```python
from build123d import *

# Parameters (mm, degrees)
SKETCH1_W                      = 1625.6
SKETCH1_H                      = 63.5
BASE_FLANGE1_DEPTH             = 1.89738
EDGE_FLANGE1_STRIP_W           = 12.66952
EDGE_FLANGE1_STRIP_H           = 1.89738
EDGE_FLANGE1_STRIP_CUT_DEPTH   = 1625.6
EDGE_FLANGE1_STRIP_2_W         = 12.66952
EDGE_FLANGE1_STRIP_2_H         = 1.89738
EDGE_FLANGE1_STRIP_CUT_2_DEPTH = 1625.6
EDGE_FLANGE1_DEPTH             = 1625.6
EDGE_FLANGE1_BEND_DEPTH        = 1625.6
SKETCH15_W                     = 9.525
SKETCH15_H                     = 50.8
CUT_EXTRUDE2_DEPTH             = 4.7752
LPATTERN3_COUNT                = 4
LPATTERN3_PITCH                = 457.2
SKETCH16_R                     = 3.3655
CUT_EXTRUDE3_DEPTH             = 2.54
LPATTERN4_COUNT                = 3
LPATTERN4_PITCH                = 762
CUT_EXTRUDE4_DEPTH             = 2.54
LPATTERN5_COUNT                = 2
LPATTERN5_PITCH                = 736.6
SKETCH18_R                     = 2.4638
CUT_EXTRUDE5_DEPTH             = 1628.038035818
SKETCH19_R                     = 2.4638
CUT_EXTRUDE6_DEPTH             = 1628.038035818
CHAMFER1_SIZE                  = 2.54


# Sheet-metal steps are written as plain solids
with BuildPart() as part:
    # Sketch1 → Base-Flange1 (new body)
    with BuildSketch(Plane(origin=(0, 0, 0), x_dir=(0, 0, -1), z_dir=(1, 0, 0))):
        with Locations((812.8, 31.75)):
            Rectangle(SKETCH1_W, SKETCH1_H)
    extrude(amount=-BASE_FLANGE1_DEPTH)

    # Edge-Flange1 strip (across the edge) → Edge-Flange1 strip cut (cut)
    with BuildSketch(Plane(origin=(-1.89738, 63.5, 0), x_dir=(0, -1, 0), z_dir=(0, 0, -1))):
        with Locations((-1.89738, -0.94869)):
            Rectangle(EDGE_FLANGE1_STRIP_W, EDGE_FLANGE1_STRIP_H)
    extrude(amount=EDGE_FLANGE1_STRIP_CUT_DEPTH, mode=Mode.SUBTRACT)

    # Edge-Flange1 strip 2 (across the edge) → Edge-Flange1 strip cut 2 (cut)
    with BuildSketch(Plane(origin=(-1.89738, 0, -1625.6), x_dir=(0, 1, 0), z_dir=(0, 0, 1))):
        with Locations((-1.89738, -0.94869)):
            Rectangle(EDGE_FLANGE1_STRIP_2_W, EDGE_FLANGE1_STRIP_2_H)
    extrude(amount=EDGE_FLANGE1_STRIP_CUT_2_DEPTH, mode=Mode.SUBTRACT)

    # Edge-Flange1 section (across the edge) → Edge-Flange1 (add)
    with BuildSketch(Plane(origin=(-1.89738, 63.5, 0), x_dir=(0, -1, 0), z_dir=(0, 0, -1))):
        with BuildLine():
            Line((0, 2.54), (0, 23.50262))
            Line((0, 23.50262), (1.89738, 23.50262))
            Line((1.89738, 23.50262), (1.89738, 2.54))
            ThreePointArc((1.89738, 2.54), (2.641328776, 0.743948776), (4.43738, 0))
            Line((4.43738, 0), (4.43738, -1.89738))
            ThreePointArc((4.43738, -1.89738), (1.299678511, -0.597701489), (0, 2.54))
        make_face()
    extrude(amount=EDGE_FLANGE1_DEPTH)

    # Edge-Flange1 section 2 (across the edge) → Edge-Flange1 bend (add)
    with BuildSketch(Plane(origin=(-1.89738, 0, -1625.6), x_dir=(0, 1, 0), z_dir=(0, 0, 1))):
        with BuildLine():
            Line((0, 2.54), (0, 23.50262))
            Line((0, 23.50262), (1.89738, 23.50262))
            Line((1.89738, 23.50262), (1.89738, 2.54))
            ThreePointArc((1.89738, 2.54), (2.641328776, 0.743948776), (4.43738, 0))
            Line((4.43738, 0), (4.43738, -1.89738))
            ThreePointArc((4.43738, -1.89738), (1.299678511, -0.597701489), (0, 2.54))
        make_face()
    extrude(amount=EDGE_FLANGE1_BEND_DEPTH)

    # Sketch15 → Cut-Extrude2 (cut)
    with BuildSketch(Plane(origin=(0, 63.5, 0), x_dir=(1, 0, 0), z_dir=(0, 1, 0))):
        with Locations((-4.7625, 127)):
            Rectangle(SKETCH15_W, SKETCH15_H)
    cut_extrude2 = extrude(amount=-CUT_EXTRUDE2_DEPTH, mode=Mode.SUBTRACT)

    # LPattern3: Cut-Extrude2 ×4
    with Locations(*[(0, 0, -i * LPATTERN3_PITCH) for i in range(1, LPATTERN3_COUNT)]):
        add(cut_extrude2, mode=Mode.SUBTRACT)

    # Sketch16 → Cut-Extrude3 (cut)
    with BuildSketch(Plane(origin=(0, 63.5, 0), x_dir=(1, 0, 0), z_dir=(0, 1, 0))):
        with Locations(Location((-12.7, 1574.8, 0), (0, 0, 180))):
            Circle(SKETCH16_R)
    cut_extrude3 = extrude(amount=-CUT_EXTRUDE3_DEPTH, mode=Mode.SUBTRACT)

    # LPattern4: Cut-Extrude3 ×3
    with Locations(*[(0, 0, i * LPATTERN4_PITCH) for i in range(1, LPATTERN4_COUNT)]):
        add(cut_extrude3, mode=Mode.SUBTRACT)

    # Sketch17 → Cut-Extrude4 (cut)
    with BuildSketch(Plane(origin=(0, 0, 0), x_dir=(0, 0, -1), z_dir=(1, 0, 0))):
        with BuildLine():
            Line((381, 47.625), (508, 47.625))
            ThreePointArc((508, 47.625), (523.875, 31.75), (508, 15.875))
            Line((508, 15.875), (381, 15.875))
            ThreePointArc((381, 15.875), (365.125, 31.75), (381, 47.625))
        make_face()
    cut_extrude4 = extrude(amount=-CUT_EXTRUDE4_DEPTH, mode=Mode.SUBTRACT)

    # LPattern5: Cut-Extrude4 ×2
    with Locations(*[(0, 0, -i * LPATTERN5_PITCH) for i in range(1, LPATTERN5_COUNT)]):
        add(cut_extrude4, mode=Mode.SUBTRACT)

    # Sketch18 → Cut-Extrude5 (cut, through all)
    with BuildSketch(Plane(origin=(0, 0, 0), x_dir=(0, 0, -1), z_dir=(1, 0, 0))):
        with Locations((546.1, 50.8)):
            Circle(SKETCH18_R)
        with Locations((546.1, 12.7)):
            Circle(SKETCH18_R)
    cut_extrude5 = extrude(amount=-CUT_EXTRUDE5_DEPTH, mode=Mode.SUBTRACT)

    # Sketch19 → Cut-Extrude6 (cut, through all)
    with BuildSketch(Plane(origin=(0, 0, 0), x_dir=(0, 0, -1), z_dir=(1, 0, 0))):
        with Locations((12.7, 50.8)):
            Circle(SKETCH19_R)
        with Locations((12.7, 12.7)):
            Circle(SKETCH19_R)
    cut_extrude6 = extrude(amount=-CUT_EXTRUDE6_DEPTH, mode=Mode.SUBTRACT)

    # Mirror1: Cut-Extrude5, Cut-Extrude6 across plane
    add(cut_extrude5.mirror(Plane.XY.offset(-812.8)), mode=Mode.SUBTRACT)
    add(cut_extrude6.mirror(Plane.XY.offset(-812.8)), mode=Mode.SUBTRACT)

    # Chamfer1
    chamfer1_edges = [part.edges().sort_by_distance(p)[0] for p in [
        (-25.4, 62.55131, 0),
        (-25.4, 62.55131, -1625.6),
        (-25.4, 0.94869, -1625.6),
        (-25.4, 0.94869, 0),
    ]]
    chamfer(chamfer1_edges, length=CHAMFER1_SIZE)


solid = part.part
```
Model file for the job. Use its own axes, mm. Give positions to 0.01 mm unless a question says otherwise; leave off trailing zeros. Loops run counter-clockwise (first coordinate to the right, second up) from the corner with the lowest first, then second, coordinate; pieces in that order, holes last. Notation, with made-up numbers: (43, 12) - (80, 12) arc R17 cw to (80, 26) - close; hole circle Ø3 at (-19.75, 2.25). An arc over 180 degrees is marked (long way). One line per item, written item: value. Start each with the question number.
1. Probe L1, parallel to Z at x = -12.7, y = 62.65; L2, parallel to Y at x = -23.25, z = -603; L3, parallel to Y at x = -0.5, z = -546.1. List the from-to ranges inside material, lowest first. Write a range as from..to.
2. Pin check, flat tips, straight feed: pin 1 (10 mm diameter, centred on y = 9.5, z = -179.5, fed in from -X); pin 2 (1.5 mm diameter, centred on x = -1, z = -1030, fed in from +Y); pin 3 (0.9 mm diameter, centred on y = 62.5, z = -126, fed in from +X) (3 decimals). Stop position of each tip, or through.
3. Pull direction Y, two halves, no side cores. Call faces 1 (the flat face through (-1.897, 32, -801)), 2 (the flat face through (0, 32, -801)): pulls with the +Y half, pulls with the -Y half, needs draft (parallel to the pull), parting line crosses it, or undercut.
4. Slice it at C-C (z = -958). List the corners of the cut face in (x, y), plus the area to 3 significant figures.
5. Slice it at A-A (z = -590). List the corners of the cut face in (x, y) (3 decimals), plus the area to 3 significant figures.
6. Slice it at B-B (y = 31.75). List the corners of the cut face in (x, z) (3 decimals), plus the area to 3 significant figures.
Solution:
1. L1: z = -1625.6..-1578.17, -1571.43..-816.17, -809.43..-54.17, -47.43..0
1. L2: y = 0..1.9, 61.6..63.5
1. L3: y = 2.39..10.24, 15.16..48.34, 53.26..61.11
2. pin 1: stops at x = -1.9
2. pin 2: stops at y = 58.72
2. pin 3: stops at x = -9.525
3. face 1: undercut
3. face 2: needs draft
4. outline: (-25.4, 0) - (-4.44, 0) arc R4.44 ccw to (0, 4.44) - (0, 59.06) arc R4.44 ccw to (-4.44, 63.5) - (-25.4, 63.5) - (-25.4, 61.6) - (-4.44, 61.6) arc R2.54 cw to (-1.9, 59.06) - (-1.9, 4.44) arc R2.54 cw to (-4.44, 1.9) - (-25.4, 1.9) - close
4. area: 204 mm^2
5. outline: (-25.4, 0) - (-4.437, 0) arc R4.437 ccw to (0, 4.437) - (0, 58.725) - (-1.897, 58.725) - (-1.897, 4.437) arc R2.54 cw to (-4.437, 1.897) - (-25.4, 1.897) - close; (-25.4, 61.603) - (-9.525, 61.603) - (-9.525, 63.5) - (-25.4, 63.5) - close
5. area: 183 mm^2
6. outline: (-1.897, -1625.6) - (0, -1625.6) - (0, -1260.475) - (-1.897, -1260.475) - close; (-1.897, -1101.725) - (0, -1101.725) - (0, -523.875) - (-1.897, -523.875) - close; (-1.897, -365.125) - (0, -365.125) - (0, 0) - (-1.897, 0) - close
6. area: 2,480 mm^2
